```python
from build123d import *

# Parameters (mm, degrees)
LOFT1_OUTLINE_W     = 5.953125
LOFT1_OUTLINE_H     = 10.31875
SKETCH5_R           = 5.969
BOSS_EXTRUDE1_DEPTH = 0.254
CUT_EXTRUDE1_DEPTH  = 0.254


with BuildPart() as part:
    # Sketch1 → Revolve1 (revolve)
    with BuildSketch(Plane(origin=(0, 0, 0), x_dir=(1, 0, 0), z_dir=(0, 1, 0)), mode=Mode.PRIVATE) as revolve1_sk:
        with BuildLine():
            Line((0, 3.571875), (0.79375, 3.571875))
            ThreePointArc((0.79375, 3.571875), (1.200596987, 4.554090513), (2.1828125, 4.9609375))
            Line((2.1828125, 4.9609375), (3.4528125, 4.9609375))
            ThreePointArc((3.4528125, 4.9609375), (4.097267114, 5.191485878), (4.449245417, 5.7785))
            Line((4.449245417, 5.7785), (10.799245417, 5.7785))
            Line((10.799245417, 5.7785), (12.77897949, 4.6355))
            Line((12.77897949, 4.6355), (14.04897949, 4.6355))
            Line((14.04897949, 4.6355), (15.36660449, 5.953125))
            Line((15.36660449, 5.953125), (28.575, 5.953125))
            Line((28.575, 5.953125), (28.575, 3.175))
            Line((28.575, 3.175), (0, 3.175))
            Line((0, 3.175), (0, 3.571875))
        make_face()
    revolve(revolve1_sk.sketch.rotate(Axis((0, 0, 0), (1, 0, 0)), 180), axis=Axis((0, 0, 0), (1, 0, 0)))

    # Loft1: read off the stored shape, not the designer's step
    # Loft1 outline → Loft1 (revolve)
    with BuildSketch(Plane.YX):
        with Locations((2.9765625, 23.415625)):
            Rectangle(LOFT1_OUTLINE_W, LOFT1_OUTLINE_H)
    revolve(axis=Axis((0, 0, 0), (1, 0, 0)))

    # Loft1 2: loft between two sections, ruled curve by curve
    loft1_2_from = [
        Edge.make_bspline([(18.25625, -7.416601563, 5.32134262), (18.25625, -7.933624268, 4.60074414), (18.25625, -8.368790825, 3.767765601), (18.25625, -8.966975982, 1.956031503), (18.25625, -9.128125, 0.978637723), (18.25625, -9.128125, -0.978637723), (18.25625, -8.966975982, -1.956031503), (18.25625, -8.368790825, -3.767765601), (18.25625, -7.933624268, -4.60074414), (18.25625, -7.416601563, -5.32134262)], [0, 0, 0, 0, 0.25, 0.25, 0.5, 0.5, 0.75, 0.75, 1, 1, 1, 1], 3),
        Edge.make_bspline([(18.25625, 7.416601563, -5.32134262), (18.25625, 7.933624268, -4.60074414), (18.25625, 8.368790825, -3.767765601), (18.25625, 8.966975982, -1.956031503), (18.25625, 9.128125, -0.978637723), (18.25625, 9.128125, 0.978637723), (18.25625, 8.966975982, 1.956031503), (18.25625, 8.368790825, 3.767765601), (18.25625, 7.933624268, 4.60074414), (18.25625, 7.416601563, 5.32134262)], [0, 0, 0, 0, 0.25, 0.25, 0.5, 0.5, 0.75, 0.75, 1, 1, 1, 1], 3),
        Edge.make_three_point_arc((18.25625, -7.416601563, -5.32134262), (18.25625, 0, -9.128125), (18.25625, 7.416601563, -5.32134262)),
        Edge.make_three_point_arc((18.25625, 7.416601563, 5.32134262), (18.25625, 0, 9.128125), (18.25625, -7.416601563, 5.32134262)),
    ]
    loft1_2_to = [
        Edge.make_bspline([(28.575, -10.31875, 7.403607123), (28.575, -10.31875, 6.169672603), (28.575, -10.31875, 4.935738082), (28.575, -10.31875, 2.467869041), (28.575, -10.31875, 1.233934521), (28.575, -10.31875, -1.233934521), (28.575, -10.31875, -2.467869041), (28.575, -10.31875, -4.935738082), (28.575, -10.31875, -6.169672603), (28.575, -10.31875, -7.403607123)], [0, 0, 0, 0, 0.25, 0.25, 0.5, 0.5, 0.75, 0.75, 1, 1, 1, 1], 3),
        Edge.make_bspline([(28.575, 10.31875, -7.403607123), (28.575, 10.31875, -6.169672603), (28.575, 10.31875, -4.935738082), (28.575, 10.31875, -2.467869041), (28.575, 10.31875, -1.233934521), (28.575, 10.31875, 1.233934521), (28.575, 10.31875, 2.467869041), (28.575, 10.31875, 4.935738082), (28.575, 10.31875, 6.169672603), (28.575, 10.31875, 7.403607123)], [0, 0, 0, 0, 0.25, 0.25, 0.5, 0.5, 0.75, 0.75, 1, 1, 1, 1], 3),
        Edge.make_three_point_arc((28.575, -10.31875, -7.403607123), (28.575, 0, -12.7), (28.575, 10.31875, -7.403607123)),
        Edge.make_three_point_arc((28.575, 10.31875, 7.403607123), (28.575, 0, 12.7), (28.575, -10.31875, 7.403607123)),
    ]
    loft1_2 = Solid(Shell([*[Face.make_surface_from_curves(loft1_2_from[k], loft1_2_to[k]) for k in range(4)], Face(Wire(loft1_2_from)), Face(Wire(loft1_2_to))]))
    add(loft1_2)

    # Sketch5 → Boss-Extrude1 (add)
    with BuildSketch(Plane(origin=(28.575, 0, 0), x_dir=(0, 0, -1), z_dir=(1, 0, 0))):
        Circle(SKETCH5_R)
    extrude(amount=BOSS_EXTRUDE1_DEPTH)

    # Sketch6 → Cut-Extrude1 (cut)
    with BuildSketch(Plane(origin=(28.829, 0, 0), x_dir=(0, 0, -1), z_dir=(1, 0, 0))):
        with BuildLine():
            Line((-3.796747786, 0.3175), (3.796747786, 0.3175))
            ThreePointArc((3.796747786, 0.3175), (0, 3.81), (-3.796747786, 0.3175))
        make_face()
        with BuildLine():
            Line((-3.796747786, -0.3175), (3.796747786, -0.3175))
            ThreePointArc((3.796747786, -0.3175), (0, -3.81), (-3.796747786, -0.3175))
        make_face()
    extrude(amount=-CUT_EXTRUDE1_DEPTH, mode=Mode.SUBTRACT)


solid = part.part
```
Source: CAD feature listing. Evaluate the final solid. Frame: model axes, mm. A direction names the side the tool comes from. Round coordinates to 2 decimals unless told otherwise and drop trailing zeros. Write each loop counter-clockwise with the first axis right and the second up, starting at its lowest first coordinate (ties: lowest second). Pieces come first, ordered by that corner, then holes. Notation, with made-up numbers: M 83,39.25 L 110,39.25 A24 ccw 110,64.25 Z; hole C 52,-22 d10. An arc over 180 degrees is marked long. Use CSV: the item, a comma, the result in double quotes. Start each with the question number.
Q1. Access query for faces 1 (the face through (28.829, 0, 0)), 2 (the face through (9, 2.8, 1.5)), 3 (the face through (28.575, 2, -6)). Directions: +Z, -Z, +X, -X, +Y, -Y. A direction counts if a zero-diameter tool reaches every point of the face in a straight line with its end or side. Return the directions, or none.
Q2. Line query: line 1 (X direction, y = 2, z = -5.75) (3 decimals); line 2 (Y direction, x = 6, z = 0) (1 decimal); line 3 (Y direction, x = 13.5, z = 0) (1 decimal). Output: solid intervals per line, ascending. Write a range as from..to.
Q3. First-contact query: P1, Ø9, axis at y = 3.5, z = 2, coming from the -X side; P2, Ø1.5, axis at x = 19, z = 9, coming from the +Y side; P3, Ø3, axis at x = 22.5, z = 9.5, coming from the +Y side; P4, Ø1, axis at y = 2.5, z = 0.5, coming from the +X side (3 decimals). Flat tips, straight axial feed; report the tip coordinate or a pass-through.
Q4. Cut plane A-A on x = 16. Output: boundary loops of the cut face in (y, z) (3 decimals), plus the area to 3 significant figures.
Q5. Pull-direction query (X, two-part tool) for faces 4 (the face through (13.42, -3.13, -3.42)), 5 (the face through (0.4, -0.16, -3.57)), 6 (the face through (28.575, -2, 0)); classes: +X half, -X half, draft (parallel to the pull), parting line (faces both ways), or undercut.
Results found:
1,face 1,"+Z, -Z, +X, +Y, -Y"
1,face 2,"-X"
1,face 3,"+X"
2,line 1,"18.256..28.575"
2,line 2,"-5.8..-3.2, 3.2..5.8"
2,line 3,"-4.6..-3.2, 3.2..4.6"
3,P1,"x = 0"
3,P2,"y = 4.58"
3,P3,"y = 7.12"
3,P4,"x = 28.575"
4,outline,"C 0,0 d11.906; hole C 0,0 d6.35"
4,area,"79.7 mm^2"
5,face 4,"undercut"
5,face 5,"draft"
5,face 6,"+X half"
